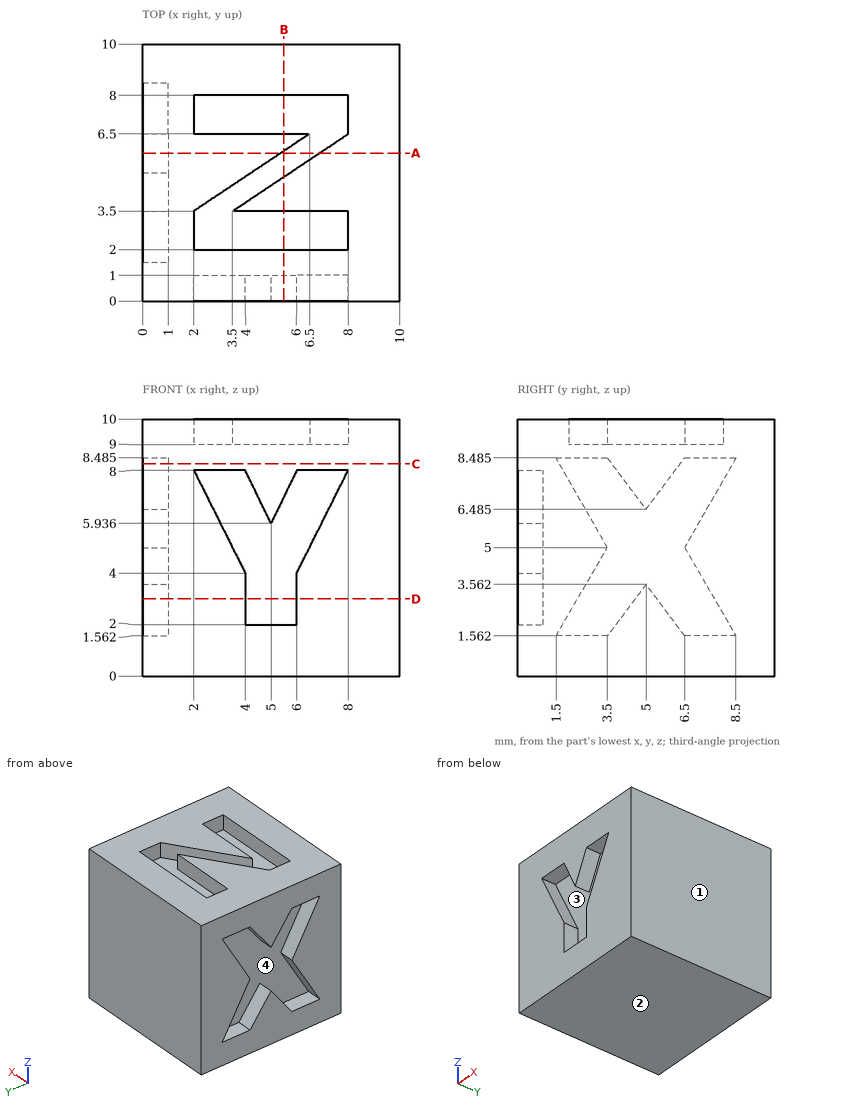
Check sheet for the drawn part. Datum: minimum x, y, z corner. Units: mm. Round coordinates to 2 decimals unless told otherwise and drop trailing zeros. Order: outer loops, then holes, each group sorted by start corner. A loop starts at its lowest first (then second) coordinate and runs counter-clockwise, first axis right, second up.
1) Scan lines: line 1 (Z direction, x = 4.75, y = 6.75); line 2 (X direction, y = 6.75, z = 2.75). Record each from-to range of solid material in increasing order.
2) Section check C-C (z = 8.25). Record the boundary of the cut face in (x, y) (1 decimal).
3) Section check A-A (y = 5.75). Record the boundary of the cut face in (x, z) (1 decimal), and give its area (3 significant figures).
4) Mould release check, pull along Z, two halves, no side actions. Record for the marked faces 1, 2, 3 and 4: +Z half, -Z half, draft (parallel to the pull), parting line (faces both ways), or undercut.
5) Section check B-B (x = 5.5). Record the boundary of the cut face in (y, z).
6) Section check D-D (z = 3). Record the boundary of the cut face in (x, y).
Result:
1. line 1: z = 0 to 9
1. line 2: x = 1 to 10
2. outline: (0, 0) - (10, 0) - (10, 10) - (0, 10) - (0, 8.4) - (1, 8.4) - (1, 6.3) - (0, 6.3) - (0, 3.7) - (1, 3.7) - (1, 1.6) - (0, 1.6) - close
3. outline: (0, 0) - (10, 0) - (10, 10) - (6.9, 10) - (6.9, 9) - (5.4, 9) - (5.4, 10) - (0, 10) - (0, 7.5) - (1, 7.5) - (1, 2.6) - (0, 2.6) - close
3. area: 93.6 mm2
4. face 1: draft
4. face 2: -Z half
4. face 3: undercut
4. face 4: undercut
5. outline: (0, 0) - (10, 0) - (10, 10) - (8, 10) - (8, 9) - (6.5, 9) - (6.5, 10) - (5.83, 10) - (5.83, 9) - (4.83, 9) - (4.83, 10) - (3.5, 10) - (3.5, 9) - (2, 9) - (2, 10) - (0, 10) - (0, 6.97) - (1, 6.97) - (1, 2) - (0, 2) - close
6. outline: (0, 0) - (4, 0) - (4, 1) - (6, 1) - (6, 0) - (10, 0) - (10, 10) - (0, 10) - (0, 7.66) - (1, 7.66) - (1, 5.42) - (0, 5.42) - (0, 4.58) - (1, 4.58) - (1, 2.34) - (0, 2.34) - close
